Design review of the part built by this model. Coordinates are the model's own, in mm. Face numbers are marked on the shaded views. A direction names the side the tool comes from. Coordinates: 2 decimals unless noted, no trailing zeros. Loops run counter-clockwise (first coordinate to the right, second up) from the corner with the lowest first, then second, coordinate; pieces in that order, holes last. Notation, with made-up numbers: (31.25, 38) -> (53.25, 38) arc R11 ccw to (53.25, 51) -> close; hole circle Ø1 at (-38, 67). An arc over 180 degrees is marked (long way). Use one line per item in the form item = value. Start each with the question number.
1. Wall thickness on line 1 (Z direction, x = 0, y = 0.15); line 2 (Z direction, x = 0, y = 2.15); line 3 (Z direction, x = 0, y = 3.35): over which ranges is each line inside the solid? List them lowest first. Write a range as from..to.
2. For pin 1 (2 mm diameter, centred on y = 2, z = 10.5, fed in from +X); pin 2 (2 mm diameter, centred on y = 1, z = -16, fed in from +X); pin 3 (1.1 mm diameter, centred on y = 1, z = 7.5, fed in from -X), all flat-tipped, find the tip position at first contact; note any pin that passes through.
3. Consider section B-B (y = 1.75). State the section outline as (x, z) points.
4. Machinability: for the marked faces 4, 5, 6, 7 and 8, which of the approach directions +Z, -Z, +X, -X, +Y, -Y give a long, thin tool a straight path to every point of the face, cutting with its end or side? Answer none if there is none.
5. The part is to be moulded in two halves that separate along X. For the marked faces 1, 2 and 3, say which applies: released by +X, released by -X, zero draft, split by the parting line, or undercut.
6. Consider section D-D (y = 3.5). State the section outline as (x, z) points, then the cut area to 3 significant figures.
7. Consider section C-C (x = 2). State the section outline as (y, z) points.
8. Consider section A-A (x = 0). State how many separate pieces and enclosed holes the cut face has, then the cut area to 3 significant figures.
Autodesk Inventor part; units mm, degrees
ref_plane "YZ Plane" through (0, 0, 0) normal (1, 0, 0) x (0, 1, 0)
ref_plane "XZ Plane" through (0, 0, 0) normal (0, 1, 0) x (-1, 0, 0)
ref_plane "XY Plane" through (0, 0, 0) normal (0, 0, 1) x (1, 0, 0)
sketch "Sketch1" plane through (0, 0, 0) normal (0, 1, 0) x (-1, 0, 0)
  circle A0 centre (0, 0) radius 1.5
  circle A1 centre (0, 0) radius 5.5
  circle A2 centre (0, -18) radius 5
  line L0 (5.4979, -0.1528) -> (4.9981, -18.1389)
  line L1 (-4.9981, -18.1389) -> (-5.4979, -0.1528)
  line L2 (0, 0) -> (0, 15) construction
  line L3 (-4, 0) -> (-4, 15)
  line L4 (4, 15) -> (4, 0)
  arc A3 (-4, 0) -> (4, 0) centre (0, 0) ccw
  arc A4 (4, 15) -> (-4, 15) centre (0, 15) ccw
  arc A5 (4, 7.5) -> (5.0769, 2.1154) centre (18, 7.5) ccw
  arc A6 (-5.0769, 2.1154) -> (-4, 7.5) centre (-18, 7.5) ccw
  point P0 (0, 7.5)
  point P1 (-4, 3.7749)
  point P2 (4, 3.7749)
  point P3 (-4, 7.5)
  dimension "d0" = 3
  dimension "d1" = 11
  dimension "d3" = 18
  dimension "d43" = 15
  dimension "d44" = 4
  dimension "d74" = 10
extrude "Extrusion1" add sketch "Sketch1" along normal blind 4
sketch "Sketch2" plane through (0, 4, 0) normal (0, 1, 0) x (1, 0, 0)
  arc A0 (4.9981, 18.1389) -> (-4.9981, 18.1389) centre (0, 18) ccw
  circle A1 centre (0, 0) radius 1.5
  line L0 (0, 16.4) -> (0, 12) construction
  line L1 (-2.6, 16.4) -> (-2.6, 12)
  line L2 (2.6, 12) -> (2.6, 16.4)
  arc A2 (2.6, 16.4) -> (-2.6, 16.4) centre (0, 16.4) ccw
  arc A3 (-2.6, 12) -> (2.6, 12) centre (0, 12) ccw
  line L3 (-4, -7.5) -> (-4, -15)
  arc A4 (-4, -15) -> (4, -15) centre (0, -15) ccw
  line L4 (4, -15) -> (4, -7.5)
  line L5 (-4.9981, 18.1389) -> (-5.4979, 0.1528)
  arc A5 (-5.4979, 0.1528) -> (-5.0769, -2.1154) centre (0, 0) ccw
  arc A6 (5.0769, -2.1154) -> (5.4979, 0.1528) centre (0, 0) ccw
  line L6 (5.4979, 0.1528) -> (4.9981, 18.1389)
  arc A7 (-4, -7.5) -> (-5.0769, -2.1154) centre (-18, -7.5) ccw
  arc A8 (5.0769, -2.1154) -> (4, -7.5) centre (18, -7.5) ccw
  point P0 (0, 14.2)
  dimension "d6" = 4.4
  dimension "d7" = 5.2
  dimension "d9" = 12
extrude "Extrusion2" cut sketch "Sketch2" against normal through all contours A2 L2 A3 L1
sketch "Sketch8" plane through (0, 4, 0) normal (0, 1, 0) x (1, 0, 0)
  line L0 (0, 31.4) -> (0, -27.4)
  line L1 (0, -14.5) -> (0, -7) construction
  line L2 (2.6, -14.5) -> (2.6, -7)
  line L3 (-2.6, -7) -> (-2.6, -14.5)
  arc A0 (-2.6, -14.5) -> (2.6, -14.5) centre (0, -14.5) ccw
  arc A1 (2.6, -7) -> (-2.6, -7) centre (0, -7) ccw
  point P0 (0, 0)
  point P1 (0, -10.75)
  dimension "d45" = 5.2
  dimension "d47" = 7
  dimension "d48" = 14.5
extrude "Extrusion8" cut sketch "Sketch8" against normal blind 1
sketch "Sketch10" plane through (0, 0, 0) normal (0, -1, 0) x (1, 0, 0)
  line L0 (0, 6.8) -> (0, 8.2) construction
  line L1 (1.1, 6.8) -> (1.1, 8.2)
  line L2 (-1.1, 8.2) -> (-1.1, 6.8)
  arc A0 (-1.1, 6.8) -> (1.1, 6.8) centre (0, 6.8) ccw
  arc A1 (1.1, 8.2) -> (-1.1, 8.2) centre (0, 8.2) ccw
  line L3 (0, 13) -> (0, 14.5) construction
  line L4 (1.1, 13) -> (1.1, 14.5)
  line L5 (-1.1, 14.5) -> (-1.1, 13)
  arc A2 (-1.1, 13) -> (1.1, 13) centre (0, 13) ccw
  arc A3 (1.1, 14.5) -> (-1.1, 14.5) centre (0, 14.5) ccw
  line L6 (0, -7.3) -> (0, -7.7) construction
  line L7 (1.1, -7.3) -> (1.1, -7.7)
  line L8 (-1.1, -7.7) -> (-1.1, -7.3)
  arc A4 (1.1, -7.3) -> (-1.1, -7.3) centre (0, -7.3) ccw
  arc A5 (-1.1, -7.7) -> (1.1, -7.7) centre (0, -7.7) ccw
  point P0 (0, 0)
  point P1 (0, 7.5)
  point P2 (0, 13.75)
  point P3 (0, -7.5)
  dimension "d60" = 2.2
  dimension "d61" = 6.8
  dimension "d62" = 1.4
  dimension "d63" = 1.5
  dimension "d64" = 2.2
  dimension "d65" = 13
  dimension "d78" = 0.2
  dimension "d79" = 7.5
extrude "Extrusion9" cut sketch "Sketch10" against normal through all contours A0 L2 A1 L1 | A2 L5 A3 L4
sketch "Sketch11" plane through (0, 0, 0) normal (0, -1, 0) x (1, 0, 0)
  circle A0 centre (0, 0) radius 4.25
  dimension "d73" = 8.5
extrude "Extrusion10" cut sketch "Sketch11" against normal blind 0.4
sketch "Sketch12" plane through (0, 4, 0) normal (0, 1, 0) x (1, 0, 0)
  circle A0 centre (0, 0) radius 2.5
  dimension "d75" = 5
extrude "Extrusion11" cut sketch "Sketch12" against normal blind 1
properties part number "Servo steering actuator v2"
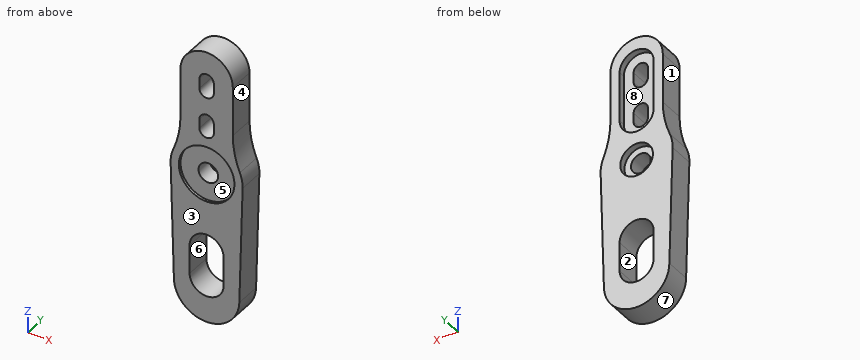
Geometry check:
q1.line_1 = -23..-19, -9.4..-4.25, 4.25..5.7, 9.3..11.9, 15.6..19
q1.line_2 = -23..-19, -9.4..-1.5, 1.5..5.7, 9.3..11.9, 15.6..19
q1.line_3 = -23..-19, -9.4..-2.5, 2.5..4.4, 17.1..19
q2.pin_1 = 4
q2.pin_2 = 5.09
q2.pin_3 = -4.01
q3.outline = (-5.5, -0.15) -> (-5, -18) arc R5 ccw to (5, -18.14) -> (5.5, -0.15) arc R5.5 ccw to (5.08, 2.12) arc R14 cw to (4, 7.5) -> (4, 15) arc R4 ccw to (-4, 15) -> (-4, 7.5) arc R14 cw to (-5.08, 2.12) arc R5.5 ccw to start; hole (-2.6, -16.4) arc R2.6 ccw to (2.6, -16.4) -> (2.6, -12) arc R2.6 ccw to (-2.6, -12) -> close; hole circle Ø3 at (0, 0); hole (-1.1, 6.8) arc R1.1 ccw to (1.1, 6.8) -> (1.1, 8.2) arc R1.1 ccw to (-1.1, 8.2) -> close; hole (-1.1, 13) arc R1.1 ccw to (1.1, 13) -> (1.1, 14.5) arc R1.1 ccw to (-1.1, 14.5) -> close
q4.face_4 = +Z, +X, +Y, -Y
q4.face_5 = -Y
q4.face_6 = +Y, -Y
q4.face_7 = -Z, +Y, -Y
q4.face_8 = +Y
q5.face_1 = released by -X
q5.face_2 = undercut
q5.face_3 = zero draft
q6.outline = (-5.5, -0.15) -> (-5, -18) arc R5 ccw to (5, -18.14) -> (5.5, -0.15) arc R5.5 ccw to (5.08, 2.12) arc R14 cw to (4, 7.5) -> (4, 15) arc R4 ccw to (-4, 15) -> (-4, 7.5) arc R14 cw to (-5.08, 2.12) arc R5.5 ccw to start; hole (-2.6, -16.4) arc R2.6 ccw to (2.6, -16.4) -> (2.6, -12) arc R2.6 ccw to (-2.6, -12) -> close; hole (-2.6, 7) arc R2.6 ccw to (2.6, 7) -> (2.6, 14.5) arc R2.6 ccw to (-2.6, 14.5) -> close; hole circle Ø5 at (0, 0)
q6.area = 259 mm²
q7.outline = (0, -22.58) -> (4, -22.58) -> (4, -18.06) -> (0, -18.06) -> close; (0, -10.34) -> (4, -10.34) -> (4, -1.5) -> (3, -1.5) -> (3, 1.5) -> (4, 1.5) -> (4, 5.34) -> (3, 5.34) -> (3, 16.16) -> (4, 16.16) -> (4, 18.46) -> (0, 18.46) -> (0, 3.75) -> (0.4, 3.75) -> (0.4, -3.75) -> (0, -3.75) -> close
q8.separate_pieces = 5
q8.enclosed_holes = 0
q8.area = 78.8 mm²
